The model under review builds one solid part; all positions refer to its coordinate system, in mm. A direction names the side the tool comes from. Coordinates: 2 decimals unless noted, no trailing zeros. Order: outer loops, then holes, each group sorted by start corner. A loop starts at its lowest first (then second) coordinate and runs counter-clockwise, first axis right, second up.
Autodesk Inventor part; units mm, degrees
ref_plane "YZ Plane" through (0, 0, 0) normal (1, 0, 0) x (0, 1, 0)
ref_plane "XZ Plane" through (0, 0, 0) normal (0, 1, 0) x (-1, 0, 0)
ref_plane "XY Plane" through (0, 0, 0) normal (0, 0, 1) x (1, 0, 0)
sketch "Sketch1" plane through (0, 0, 0) normal (0, 0, 1) x (1, 0, 0)
  line L0 (-150, 74.8538) -> (150, 74.8538)
  line L1 (150, 74.8538) -> (150, -225.1462)
  line L2 (150, -225.1462) -> (-150, -225.1462)
  line L3 (-150, -225.1462) -> (-150, 74.8538)
  point P0 (0, 0)
  dimension "d0" = 300
  dimension "d1" = 300
  dimension "d2" = 150
extrude "Extrusion1" add sketch "Sketch1" along normal blind 100
shell "Shell1" thickness 10 removed faces 1 at (-50, -25.1462, 100)
sketch "Sketch2" plane through (-140, 64.8538, 10) normal (0, 0, 1) x (1, 0, 0)
  circle A0 centre (140, -178.7412) radius 35
  circle A1 centre (140, -178.7412) radius 35
  circle A2 centre (140, -178.7412) radius 35
  point P0 (140, -64.8538)
extrude "Extrusion2" cut sketch "Sketch2" against normal up to next
sketch "Sketch3" plane through (0, 0, 100) normal (0, 0, 1) x (1, 0, 0)
  line L0 (-140, 64.8538) -> (140, 64.8538)
  line L1 (-150, 74.8538) -> (-150, -225.1462)
  line L2 (150, -225.1462) -> (150, 74.8538)
  line L3 (140, -215.1462) -> (-140, -215.1462)
  point P0 (0, 0)
  point P1 (-144, 68.8538)
  point P2 (144, 68.8538)
  point P3 (144, -219.1462)
  point P4 (-144, -219.1462)
  dimension "d8" = 4
  dimension "d9" = 6
  dimension "d10" = 6
  dimension "d11" = 6
  dimension "d12" = 6
  dimension "d13" = 4
  dimension "d14" = 4
  dimension "d15" = 4
hole "Hole1" at (-144, 68.8538, 100) at (144, 68.8538, 100) at (144, -219.1462, 100) at (-144, -219.1462, 100) direction (0, 0, -1) diameter 6.647 depth 22.2 tip angle 118
properties part number "aanstuurkast"
(1) Consider section D-D (x = -97). Give the boundary of the cut face in (y, z), then the cut area to 3 significant figures.
(2) The part is to be moulded in two halves that separate along X. For faces 3 (the face through (-143.83, -219.7, 76.15)), 4 (the face through (-1, 70, 100)), 5 (the face through (150, -73, 49)), say which applies: +X half, -X half, draft (parallel to the pull), parting line (faces both ways), or undercut.
(3) Consider section B-B (z = 54). Give the boundary of the cut face in (x, y), then the cut area to 3 significant figures.
(4) Wall thickness on line 1 (Y direction, x = -144, z = 94); line 2 (X direction, y = -29.5, z = 42.5); line 3 (Y direction, x = -101, z = 21.5): over which ranges is each line inside the solid? List them lowest first.
(5) Consider section C-C (y = -168.5). Give the boundary of the cut face in (x, z).
(6) Consider section A-A (x = 0). Give the boundary of the cut face in (y, z).
(7) Insertion check: pin 1 Ø12 at (x, y) = (-105, -150) entering from -Z; pin 2 Ø3 at (x, y) = (102, -170.5) entering from +Z; pin 3 Ø5.5 at (x, y) = (144, -219.15) entering from +Z. Each pin has a flat end and moves straight along its axis. Give the tip position at first contact, or say it passes through.
(8) Tool access review of faces 1 (the face through (-25.796, -90.233, 5.07)), 2 (the face through (-2, 64.854, 54)): name each direction out of +Z, -Z, +X, -X, +Y, -Y from which nothing blocks a thin tool from reaching the whole face with its end or side.
Findings:
1. outline: (-225.15, 0) - (74.85, 0) - (74.85, 100) - (64.85, 100) - (64.85, 10) - (-215.15, 10) - (-215.15, 100) - (-225.15, 100) - close
1. area: 4,800 mm2
2. face 3: undercut
2. face 4: draft
2. face 5: +X half
3. outline: (-150, -225.15) - (150, -225.15) - (150, 74.85) - (-150, 74.85) - close; hole (-140, -215.15) - (140, -215.15) - (140, 64.85) - (-140, 64.85) - close
3. area: 11,600 mm2
4. line 1: y = -225.15 to -222.47, -215.82 to 65.53, 72.18 to 74.85
4. line 2: x = -150 to -140, 140 to 150
4. line 3: y = -225.15 to -215.15, 64.85 to 74.85
5. outline: (-150, 0) - (150, 0) - (150, 100) - (140, 100) - (140, 10) - (-140, 10) - (-140, 100) - (-150, 100) - close
6. outline: (-225.15, 0) - (-148.89, 0) - (-148.89, 10) - (-215.15, 10) - (-215.15, 100) - (-225.15, 100) - close; (-78.89, 0) - (74.85, 0) - (74.85, 100) - (64.85, 100) - (64.85, 10) - (-78.89, 10) - close
7. pin 1: stops at z = 0
7. pin 2: stops at z = 10
7. pin 3: stops at z = 77.46
8. face 1: +Z, -Z
8. face 2: +Z
